from build123d import *

# Parameters (mm, degrees)
SKETCH2_W           = 0.5
SKETCH2_H           = 0.5
BOSS_EXTRUDE1_DEPTH = 5
CUT_EXTRUDE1_REACH  = 10.6


with BuildPart() as part:
    # Sketch1 → Revolve3 (revolve)
    with BuildSketch(Plane(origin=(0, 0, 0), x_dir=(1, 0, 0), z_dir=(0, 1, 0))):
        with BuildLine():
            Line((0.041424419, -1.31875), (-2.908575581, -1.31875))
            Line((-2.908575581, -1.31875), (-2.908575581, -0.31875))
            Line((-2.908575581, -0.31875), (-2.458575581, -0.31875))
            Line((-2.458575581, -0.31875), (-2.458575581, 4.78125))
            ThreePointArc((-2.458575581, 4.78125), (-1.726342534, 6.549016953), (0.041424419, 7.28125))
            Line((0.041424419, 7.28125), (0.041424419, 6.960699472))
            Line((0.041424419, 6.960699472), (-0.258575581, 6.960699472))
            ThreePointArc((-0.258575581, 6.960699472), (-1.616887977, 6.226933229), (-2.158575581, 4.78125))
            Line((-2.158575581, 4.78125), (-2.158575581, -0.61875))
            Line((-2.158575581, -0.61875), (-2.608575581, -0.61875))
            Line((-2.608575581, -0.61875), (-2.608575581, -1.01875))
            Line((-2.608575581, -1.01875), (-0.258575581, -1.01875))
            Line((-0.258575581, -1.01875), (0.041424419, -1.01875))
            Line((0.041424419, -1.01875), (0.041424419, -1.31875))
        make_face()
    revolve(axis=Axis((0.041424419, 0, -7.28125), (0, 0, 1)))

    # Sketch2 → Boss-Extrude1 (add)
    with BuildSketch(Plane.XY.offset(1.31875)):
        with Locations((1.27, -0.01024953)):
            Rectangle(SKETCH2_W, SKETCH2_H)
        with Locations((-1.27, -0.01024953)):
            Rectangle(SKETCH2_W, SKETCH2_H)
    extrude(amount=BOSS_EXTRUDE1_DEPTH)

    # Sketch3 → Cut-Extrude1 (cut, up to next)
    with BuildSketch(Plane(origin=(0.020061741, 0, 1.31875), x_dir=(1, 0, 0), z_dir=(0, 0, 1)), mode=Mode.PRIVATE) as cut_extrude1_sk1:
        Polygon((2.675232006, 2.192680339), (2.675232006, -2.268878516), (4.29481628, -2.502381421), (4.160489908, 2.299424082), align=None)
    cut_extrude1_tool1 = extrude(cut_extrude1_sk1.sketch, amount=-CUT_EXTRUDE1_REACH, mode=Mode.PRIVATE) & part.part
    add(cut_extrude1_tool1.solids().sort_by_distance((3.481327, -0.10236, 1.31875))[0], mode=Mode.SUBTRACT)


solid = part.part
Input: part model. Units: mm. Frame: model coordinates. A direction names the side the tool comes from. Coordinates: 2 decimals unless noted, no trailing zeros. Loops run counter-clockwise (first coordinate to the right, second up) from the corner with the lowest first, then second, coordinate; pieces in that order, holes last. Notation, with made-up numbers: (2.25, 83.25) - (25.25, 83.25) arc R28 cw to (25.25, 102.25) - close; hole circle Ø8 at (62, 75). An arc over 180 degrees is marked (long way). Answer in a Markdown table with one row per item. Add a question column.
Item 1: Mould query, pull axis Y, two halves, no side actions, for faces 3 (the cylindrical face through (0.616, 2.587, 0.822)), 4 (the flat face through (0, 0, 1.319)), 5 (the cylindrical face through (-2.343, -0.751, -2.267)), 6 (the flat face through (0, 0, 1.019)). Classes: released by +Y, released by -Y, zero draft, split by the parting line, or undercut.
Item 2: Section query C-C on x = 1.7. Return the cut outline in (y, z), then the cut area to 3 significant figures.
Item 3: Contact query for flat-ended pins moving along their axis: P1, Ø2, axis at x = 1.5, z = -4.5, coming from the -Y side; P2, Ø1.5, axis at x = -2.5, z = -2, coming from the +Y side; P3, Ø1.7, axis at x = 0, y = -1, coming from the -Z side. Output: stop coordinate, or through.
Item 4: Section query B-B on y = 0.8. Return the cut outline in (x, z), then the cut area to 3 significant figures.
Item 5: Access query for faces 1 (the cylindrical face through (-2.906, 0.111, 0.812)), 2 (the cylindrical face through (-2.057, -0.661, -2.043)). Directions: +Z, -Z, +X, -X, +Y, -Y. A direction counts if a zero-diameter tool reaches every point of the face in a straight line with its end or side. Return the directions, or none.
Item 6: Section query D-D on z = -4. Return the cut outline in (x, y), then the cut area to 3 significant figures.
Item 7: Line query: line 1 along Z through (x, y) = (1.35, -2.2); line 2 along X through (y, z) = (0, -3.35); line 3 along X through (y, z) = (0.6, 0.5). Output: solid intervals per line, ascending. Write a range as [from, to].
Item 8: Section query A-A on z = 1.5. Return the cut outline in (x, y), then the cut area to 3 significant figures.
Recorded:
| question | item | result |
|---|---|---|
| 1 | face 3 | undercut |
| 1 | face 4 | zero draft |
| 1 | face 5 | split by the parting line |
| 1 | face 6 | undercut |
| 2 | outline | (-2.44, 0.32) - (-1.87, 0.32) - (-1.87, -4.78) arc R1.87 ccw to (1.87, -4.78) - (1.87, 0.32) - (2.44, 0.32) - (2.44, 1.32) - (-2.44, 1.32) - close; hole (-2.07, 0.62) - (-1.45, 0.62) - (-1.45, -4.78) arc R1.45 ccw to (1.45, -4.78) - (1.45, 0.62) - (2.07, 0.62) - (2.07, 1.02) - (-2.07, 1.02) - close |
| 2 | area | 8.91 mm^2 |
| 3 | P1 | y = -2.46 |
| 3 | P2 | y = 1.74 |
| 3 | P3 | z = -7.28 |
| 4 | outline | (-2.8, 0.32) - (-2.33, 0.32) - (-2.33, -4.78) arc R2.37 ccw to (2.41, -4.78) - (2.41, 0.32) - (2.7, 0.32) - (2.7, 1.32) - (-2.8, 1.32) - close; hole (-2.48, 0.62) - (-2.01, 0.62) - (-2.01, -4.78) arc R2.05 ccw to (2.09, -4.78) - (2.09, 0.62) - (2.57, 0.62) - (2.57, 1.02) - (-2.48, 1.02) - close |
| 4 | area | 7.71 mm^2 |
| 5 | face 1 | +Z, -Z |
| 5 | face 2 | none |
| 6 | outline | circle Ø5 at (0.04, 0); hole circle Ø4.4 at (0.04, 0) |
| 6 | area | 4.43 mm^2 |
| 7 | line 1 | [0.32, 0.62], [1.02, 1.32] |
| 7 | line 2 | [-2.46, -2.16], [2.24, 2.54] |
| 7 | line 3 | [-2.85, -2.08], [2.16, 2.7] |
| 8 | outline | (-1.52, -0.26) - (-1.02, -0.26) - (-1.02, 0.24) - (-1.52, 0.24) - close; (1.02, -0.26) - (1.52, -0.26) - (1.52, 0.24) - (1.02, 0.24) - close |
| 8 | area | 0.500 mm^2 |
